Geometry check sheet. Reference: the model listing, model coordinates, mm. Round coordinates to 2 decimals unless told otherwise and drop trailing zeros. Write each loop counter-clockwise with the first axis right and the second up, starting at its lowest first coordinate (ties: lowest second). Pieces come first, ordered by that corner, then holes. Notation, with made-up numbers: M -36,-16.75 L -29,-16.75 A28 cw -29,5.25 Z; hole C 16.5,-11 d6. An arc over 180 degrees is marked long. One line per item, written item: value. Start each with the question number.
1. Depth check by flat-ended pin: P1, Ø0.8, axis at x = -71, z = 1.5, coming from the -Y side; P2, Ø12, axis at x = -42.15, y = -45.34, coming from the -Z side; P3, Ø1.5, axis at y = -101, z = 1.5, coming from the +X side; P4, Ø0.8, axis at y = -92, z = 0.5, coming from the +X side. Enter the tip coordinate at first touch or a pass-through.
2. Section check A-A (x = -87.5). Record the boundary of the cut face in (y, z), and give its area (3 significant figures).
3. Section check D-D (z = 1.45). Count the separate pieces of the cut face and the enclosed holes in it, and give its area (3 significant figures).
4. Section check B-B (x = 31.5). Record the boundary of the cut face in (y, z), and give its area (3 significant figures).
5. Section check C-C (y = -33). Record the boundary of the cut face in (x, z).
6. Scan lines: probe 1 along X at (y, z) = (-52, 2.2); probe 2 along X at (y, z) = (-40, 1.6); probe 3 along Y at (x, z) = (-84.5, 1.85). Record each from-to range of solid material in increasing order. Write a range as [from, to].
from build123d import *

# Parameters (mm, degrees)
SKETCH1_W           = 160
SKETCH1_H           = 90
BOSS_EXTRUDE8_DEPTH = 3
FILLET15_R          = 5
FILLET16_R          = 5
SKETCH14_R          = 10
SKETCH14_R_2        = 2
SKETCH14_W          = 7.5
SKETCH14_H          = 6
SKETCH14_W_2        = 6
SKETCH14_H_2        = 10
CUT_EXTRUDE1_DEPTH  = 3
FILLET17_R          = 0.5


with BuildPart() as part:
    # Sketch1 → Boss-Extrude8 (new body)
    with BuildSketch(Plane.XY):
        with Locations((-31.627906977, -65.930232558)):
            Rectangle(SKETCH1_W, SKETCH1_H)
    extrude(amount=BOSS_EXTRUDE8_DEPTH)

    # Fillet15
    fillet15_edges = [part.edges().sort_by_distance(p)[0] for p in [
        (-111.627906977, -20.930232558, 1.5),
        (48.372093023, -20.930232558, 1.5),
        (48.372093023, -110.930232558, 1.5),
        (-111.627906977, -110.930232558, 1.5),
    ]]
    fillet(fillet15_edges, radius=FILLET15_R)

    # Fillet16
    # the kernel refuses this fillet: 5 mm, written as the material it takes off along each edge
    with BuildSketch(Plane(origin=(-106.627906977, -25.930232558, 3), x_dir=(0, 1, 0), z_dir=(1, 0, 0))) as fillet16_piece_1:
        with BuildLine():
            CenterArc((0.417424305, -5), FILLET16_R, 23.578178478, 66.421821522)
            Line((0.417424305, 0), (0.417424305, 0.1))
            Line((0.417424305, 0.1), (5, 0.1))
            Line((5, 0.1), (5.1, 0))
            ThreePointArc((5.1, 0), (5.1, -1.5), (5.091651514, -2.96))
            Line((5.091651514, -2.96), (5, -3))
        make_face()
    revolve(axis=Axis((-106.627906977, -25.930232558, 3), (0, 0, 1)), revolution_arc=90, mode=Mode.SUBTRACT)
    with BuildSketch(Plane(origin=(-106.627906977, -20.930232558, 3), x_dir=(0, 0, -1), z_dir=(1, 0, 0))) as fillet16_piece_2:
        with BuildLine():
            CenterArc((5, -4.582575695), FILLET16_R, 113.578178478, 66.421821522)
            Line((0, -4.582575695), (-0.1, -4.582575695))
            Line((-0.1, -4.582575695), (-0.1, 0))
            Line((-0.1, 0), (0, 0.1))
            ThreePointArc((0, 0.1), (1.5, 0.1), (2.96, 0.091651514))
            Line((2.96, 0.091651514), (3, 0))
        make_face()
    extrude(amount=150, mode=Mode.SUBTRACT)
    with BuildSketch(Plane(origin=(43.372093023, -25.930232558, 3), x_dir=(0, 1, 0), z_dir=(-1, 0, 0))) as fillet16_piece_3:
        with BuildLine():
            CenterArc((0.417424305, 5), FILLET16_R, 270, 66.421821522)
            Line((0.417424305, 0), (0.417424305, -0.1))
            Line((0.417424305, -0.1), (5, -0.1))
            Line((5, -0.1), (5.1, 0))
            ThreePointArc((5.1, 0), (5.1, 1.5), (5.091651514, 2.96))
            Line((5.091651514, 2.96), (5, 3))
        make_face()
    revolve(axis=Axis((43.372093023, -25.930232558, 3), (0, 0, -1)), revolution_arc=90, mode=Mode.SUBTRACT)
    with BuildSketch(Plane(origin=(48.372093023, -25.930232558, 3), x_dir=(-1, 0, 0), z_dir=(0, -1, 0)), Plane(origin=(-111.627906977, -105.930232558, 3), x_dir=(1, 0, 0), z_dir=(0, 1, 0))) as fillet16_piece_4:
        with BuildLine():
            CenterArc((4.582575695, 5), FILLET16_R, 203.578178478, 66.421821522)
            Line((0, 3), (-0.091651514, 2.96))
            ThreePointArc((-0.091651514, 2.96), (-0.1, 1.5), (-0.1, 0))
            Line((-0.1, 0), (0, -0.1))
            Line((0, -0.1), (4.582575695, -0.1))
            Line((4.582575695, -0.1), (4.582575695, 0))
        make_face()
    extrude(amount=80, mode=Mode.SUBTRACT)
    with BuildSketch(Plane(origin=(43.372093023, -105.930232558, 3), x_dir=(1, 0, 0), z_dir=(0, 1, 0))) as fillet16_piece_5:
        with BuildLine():
            CenterArc((0.417424305, 5), FILLET16_R, 270, 66.421821522)
            Line((5, 3), (5.091651514, 2.96))
            ThreePointArc((5.091651514, 2.96), (5.1, 1.5), (5.1, 0))
            Line((5.1, 0), (5, -0.1))
            Line((5, -0.1), (0.417424305, -0.1))
            Line((0.417424305, -0.1), (0.417424305, 0))
        make_face()
    revolve(axis=Axis((43.372093023, -105.930232558, 3), (0, 0, -1)), revolution_arc=90, mode=Mode.SUBTRACT)
    with BuildSketch(Plane(origin=(43.372093023, -110.930232558, 3), x_dir=(0, 1, 0), z_dir=(-1, 0, 0))) as fillet16_piece_6:
        with BuildLine():
            CenterArc((4.582575695, 5), FILLET16_R, 203.578178478, 66.421821522)
            Line((0, 3), (-0.091651514, 2.96))
            ThreePointArc((-0.091651514, 2.96), (-0.1, 1.5), (-0.1, 0))
            Line((-0.1, 0), (0, -0.1))
            Line((0, -0.1), (4.582575695, -0.1))
            Line((4.582575695, -0.1), (4.582575695, 0))
        make_face()
    extrude(amount=150, mode=Mode.SUBTRACT)
    with BuildSketch(Plane(origin=(-106.627906977, -105.930232558, 3), x_dir=(0, -1, 0), z_dir=(1, 0, 0))) as fillet16_piece_7:
        with BuildLine():
            CenterArc((0.417424305, 5), FILLET16_R, 270, 66.421821522)
            Line((5, 3), (5.091651514, 2.96))
            ThreePointArc((5.091651514, 2.96), (5.1, 1.5), (5.1, 0))
            Line((5.1, 0), (5, -0.1))
            Line((5, -0.1), (0.417424305, -0.1))
            Line((0.417424305, -0.1), (0.417424305, 0))
        make_face()
    revolve(axis=Axis((-106.627906977, -105.930232558, 3), (0, 0, -1)), revolution_arc=90, mode=Mode.SUBTRACT)

    # Sketch14 → Cut-Extrude1 (cut)
    with BuildSketch(Plane.XY.offset(3)):
        with Locations((-42.146770789, -45.341082591)):
            Circle(SKETCH14_R)
        with Locations((-103.87862187, -65.341099016)):
            Circle(SKETCH14_R_2)
        with Locations((40.552517345, -65.341099016)):
            Circle(SKETCH14_R_2)
        with Locations((-20.211230278, -45.387431922)):
            Circle(SKETCH14_R)
        with Locations((-57.943307222, -90.939107411)):
            Rectangle(SKETCH14_W, SKETCH14_H)
        with Locations((-71.994996652, -65.002222921)):
            Rectangle(SKETCH14_W_2, SKETCH14_H_2)
        with Locations((-87.217465232, -90.960925791)):
            Rectangle(SKETCH14_W, SKETCH14_H)
        with BuildLine():
            Line((-73.975530372, -49.539987585), (-70.259376522, -49.539987585))
            ThreePointArc((-70.259376522, -49.539987585), (-69.259376522, -50.539987585), (-70.259376522, -51.539987585))
            Line((-70.259376522, -51.539987585), (-73.975530372, -51.539987585))
            ThreePointArc((-73.975530372, -51.539987585), (-74.975530372, -50.539987585), (-73.975530372, -49.539987585))
        make_face()
        with Locations((24.261172399, -90.711648075)):
            Rectangle(SKETCH14_W, SKETCH14_H)
        with Locations((10.209482969, -64.774763585)):
            Rectangle(SKETCH14_W_2, SKETCH14_H_2)
        with Locations((-5.012985611, -90.733466455)):
            Rectangle(SKETCH14_W, SKETCH14_H)
        with BuildLine():
            Line((8.228949249, -49.312528249), (11.945103099, -49.312528249))
            ThreePointArc((11.945103099, -49.312528249), (12.945103099, -50.312528249), (11.945103099, -51.312528249))
            Line((11.945103099, -51.312528249), (8.228949249, -51.312528249))
            ThreePointArc((8.228949249, -51.312528249), (7.228949249, -50.312528249), (8.228949249, -49.312528249))
        make_face()
        with BuildLine():
            Line((-34.976059895, -59.255469081), (-28.389202639, -59.255469081))
            ThreePointArc((-28.389202639, -59.255469081), (-25.889202639, -61.755469081), (-28.389202639, -64.255469081))
            Line((-28.389202639, -64.255469081), (-34.976059895, -64.255469081))
            ThreePointArc((-34.976059895, -64.255469081), (-37.476059895, -61.755469081), (-34.976059895, -59.255469081))
        make_face()
    extrude(amount=-CUT_EXTRUDE1_DEPTH, mode=Mode.SUBTRACT)

    # Fillet17
    fillet17_edges = [part.edges().sort_by_distance(p)[0] for p in [
        (20.511172399, -90.711648075, 3),
        (24.261172399, -93.711648075, 3),
        (28.011172399, -90.711648075, 3),
        (24.261172399, -87.711648075, 3),
        (-8.762985611, -90.733466455, 3),
        (-5.012985611, -93.733466455, 3),
        (-1.262985611, -90.733466455, 3),
        (-5.012985611, -87.733466455, 3),
        (7.209482969, -64.774763585, 3),
        (10.209482969, -69.774763585, 3),
        (13.209482969, -64.774763585, 3),
        (10.209482969, -59.774763585, 3),
        (-61.693307222, -90.939107411, 3),
        (-57.943307222, -93.939107411, 3),
        (-54.193307222, -90.939107411, 3),
        (-57.943307222, -87.939107411, 3),
        (-90.967465232, -90.960925791, 3),
        (-87.217465232, -93.960925791, 3),
        (-83.467465232, -90.960925791, 3),
        (-87.217465232, -87.960925791, 3),
        (38.552517345, -65.341099016, 3),
        (-105.87862187, -65.341099016, 3),
        (-74.994996652, -65.002222921, 3),
        (-71.994996652, -70.002222921, 3),
        (-68.994996652, -65.002222921, 3),
        (-71.994996652, -60.002222921, 3),
    ]]
    fillet(fillet17_edges, radius=FILLET17_R)


solid = part.part
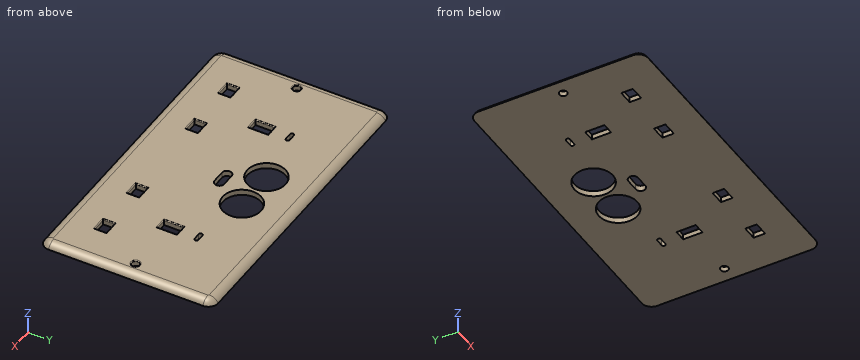
Result sheet:
1. P1: stops at y = -110.27
1. P2: passes through
1. P3: stops at x = 47.97
1. P4: stops at x = 48.33
2. outline: M -110.93,0 L -93.96,0 L -93.96,2.5 A0.5 ccw -94.46,3 L -106.35,3 A5 ccw Z; M -87.96,0 L -20.93,0 A5 ccw -25.51,3 L -87.46,3 A0.5 ccw -87.96,2.5 Z
2. area: 244 mm2
3. separate pieces: 1
3. enclosed holes: 13
3. area: 12,900 mm2
4. outline: M -110.93,0 L -20.93,0 A5 ccw -25.51,3 L -106.35,3 A5 ccw Z
4. area: 262 mm2
5. outline: M -111.63,0 L 48.37,0 A5 ccw 43.79,3 L -107.05,3 A5 ccw Z
6. probe 1: x = [-109.76, -49.61], [-34.69, -27.71], [-12.71, 46.5]
6. probe 2: x = [-110.52, -50.6], [-33.69, -28.64], [-11.79, 47.26]
6. probe 3: y = [-109.54, -93.96], [-87.96, -22.32]
